Can you work these out from the drawing? Everything is in mm from the part's minimum corner. A direction names the side the tool comes from. Give positions to 0.01 mm unless a question says otherwise; leave off trailing zeros. Write each loop counter-clockwise with the first axis right and the second up, starting at its lowest first coordinate (ties: lowest second). Pieces come first, ordered by that corner, then holes. Notation, with made-up numbers: (-8.5, -31) - (24.5, -31) arc R24 cw to (24.5, -16) - close; hole circle Ø6 at (61.25, 3.25). An arc over 180 degrees is marked (long way). Use a Markdown table: item, result.
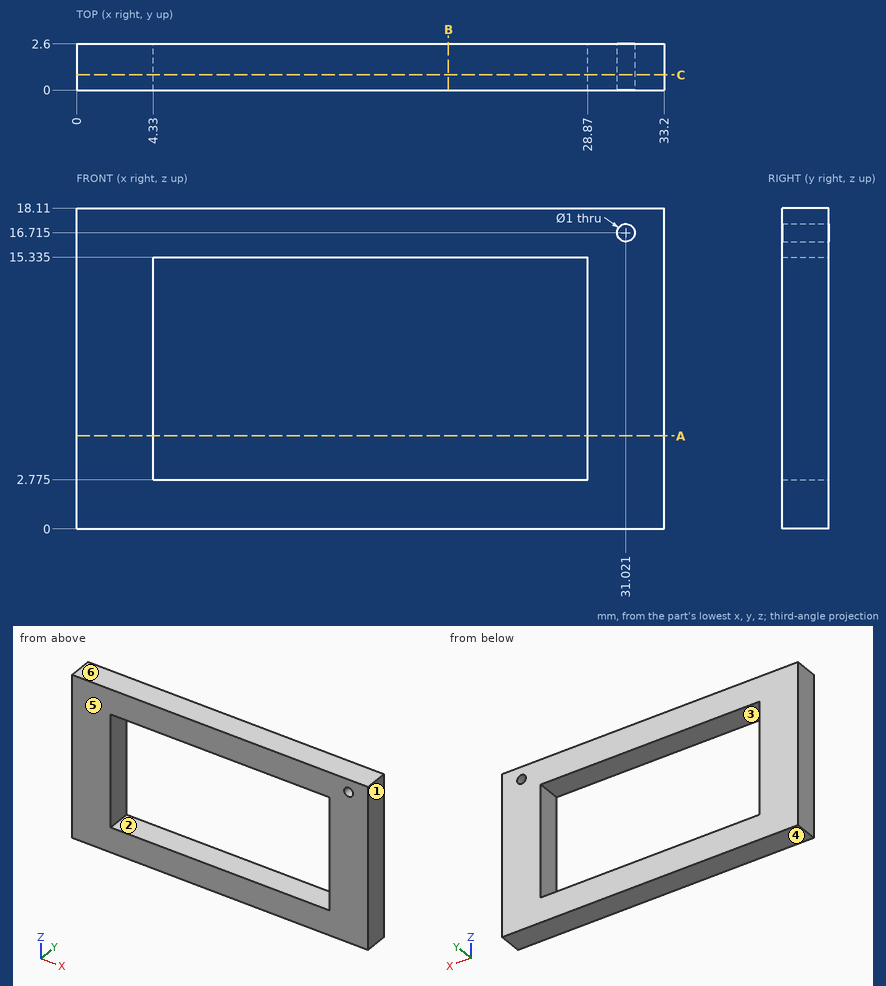
Item 1: If we section it at B-B, the plane x = 21: Write out the boundary of the cut face in (y, z) (1 decimal).
Values:
| item | result |
|---|---|
| outline | (0, 0) - (2.6, 0) - (2.6, 2.8) - (0, 2.8) - close; (0, 15.3) - (2.6, 15.3) - (2.6, 18.1) - (0, 18.1) - close |
Item 2: Thinking about a two-plate mould opening in Z: for the marked faces 3, 4, 5 and 6, which applies, +Z half, -Z half, draft (parallel to the pull), parting line (faces both ways), or undercut?
Values:
| item | result |
|---|---|
| face 3 | undercut |
| face 4 | -Z half |
| face 5 | draft |
| face 6 | +Z half |
Item 3: I need wall thicknesses on line 1 along Z through (x, y) = (21.5, 1.75) (1 decimal); line 2 along X through (y, z) = (2, 6.25); line 3 along Z through (x, y) = (31, 1) (1 decimal). Which ranges of each line are inside material? Lowest first, please. Write a range as [from, to].
Values:
| item | result |
|---|---|
| line 1 | z = [0, 2.8], [15.3, 18.1] |
| line 2 | x = [0, 4.33], [28.87, 33.2] |
| line 3 | z = [0, 16.2], [17.2, 18.1] |
Item 4: For the marked faces 1 and 2, which set-ups out of +Z, -Z, +X, -X, +Y, -Y let a thin tool reach every point of the face, with its end or its side?
Values:
| item | result |
|---|---|
| face 1 | +Z, -Z, +X, +Y, -Y |
| face 2 | +Y, -Y |
Item 5: Will this pin go through, and if not, where does the flat tip stop? pin 1 Ø1 at (x, z) = (12.5, 13) entering from +Y.
Values:
| item | result |
|---|---|
| pin 1 | passes through |
Item 6: If we section it at C-C, the plane y = 0.85: Write out the boundary of the cut face in (x, z) (1 decimal).
Values:
| item | result |
|---|---|
| outline | (0, 0) - (33.2, 0) - (33.2, 18.1) - (0, 18.1) - close; hole (4.3, 2.8) - (28.9, 2.8) - (28.9, 15.3) - (4.3, 15.3) - close; hole circle Ø1 at (31, 16.7) |
Item 7: If we section it at A-A, the plane z = 5.25: Write out the boundary of the cut face in (x, y), plus the area to 3 significant figures.
Values:
| item | result |
|---|---|
| outline | (0, 0) - (4.33, 0) - (4.33, 2.6) - (0, 2.6) - close; (28.87, 0) - (33.2, 0) - (33.2, 2.6) - (28.87, 2.6) - close |
| area | 22.5 mm2 |
